Build history of the part. All positions in model axes, mm. A direction names the side the tool comes from. Give positions to 0.01 mm unless a question says otherwise; leave off trailing zeros. Order: outer loops, then holes, each group sorted by start corner. A loop starts at its lowest first (then second) coordinate and runs counter-clockwise, first axis right, second up. Notation, with made-up numbers: (62, 65.25) -> (89, 65.25) arc R18 ccw to (89, 89.25) -> close; hole circle Ø9 at (70, 83.5). An arc over 180 degrees is marked (long way). Write item = value, one per line. Start each with the question number.
from build123d import *

# Parameters (mm, degrees)
BOSS_EXTRUDE1_DEPTH = 76.2
FILLET1_R           = 127
CUT_EXTRUDE1_DEPTH  = 152.4
SKETCH4_R           = 38.1
CUT_EXTRUDE2_DEPTH  = 152.4
SKETCH5_R           = 330.2
SKETCH5_R_2         = 279.4
BOSS_EXTRUDE2_DEPTH = 76.2
CUT_EXTRUDE3_DEPTH  = 76.2
SKETCH7_R           = 279.4
CUT_EXTRUDE4_DEPTH  = 76.2
FILLET2_R           = 101.6
SKETCH10_R          = 19.05
CUT_EXTRUDE5_DEPTH  = 1983.041579978


with BuildPart() as part:
    # Sketch1 → Boss-Extrude1 (new, symmetric)
    with BuildSketch(Plane(origin=(0, 0, 0), x_dir=(1, 0, 0), z_dir=(0, 1, 0))):
        Polygon((666.144379946, 38.507212604), (1092.864379946, -322.007837556), (1913.344533237, -322.007837556), (1913.344533237, -398.207837556), (1064.984533237, -398.207837556), (638.264533237, -37.692787396), (-652.055466763, -37.692787396), (-652.055466763, 38.507212604), align=None)
    extrude(amount=BOSS_EXTRUDE1_DEPTH, both=True)

    # Fillet1
    fillet1_edges = [part.edges().sort_by_distance(p)[0] for p in [
        (666.144379946, 0, -38.507212604),
        (1092.864379946, 0, 322.007837556),
        (1064.984533237, 0, 398.207837556),
        (638.264533237, 0, 37.692787396),
    ]]
    fillet(fillet1_edges, radius=FILLET1_R)

    # Sketch3 → Cut-Extrude1 (cut)
    with BuildSketch(Plane.XY.offset(37.692787396)):
        with BuildLine():
            ThreePointArc((-652.055466763, -4.31e-07), (-629.737003641, 53.881536574), (-575.855466763, 76.2))
            Line((-575.855466763, 76.2), (-652.055466763, 76.2))
            Line((-652.055466763, 76.2), (-652.055466763, -4.31e-07))
        make_face()
        with BuildLine():
            ThreePointArc((-575.855466763, -76.2), (-629.737003336, -53.881536879), (-652.055466763, -4.31e-07))
            Line((-652.055466763, -4.31e-07), (-652.055466763, -76.2))
            Line((-652.055466763, -76.2), (-575.855466763, -76.2))
        make_face()
    extrude(amount=-CUT_EXTRUDE1_DEPTH, mode=Mode.SUBTRACT)

    # Sketch4 → Cut-Extrude2 (cut)
    with BuildSketch(Plane.XY.offset(37.692787396)):
        with Locations((-575.855466763, 0)):
            Circle(SKETCH4_R)
    extrude(amount=-CUT_EXTRUDE2_DEPTH, mode=Mode.SUBTRACT)

    # Sketch5 → Boss-Extrude2 (add)
    with BuildSketch(Plane.XY.offset(398.207837556)):
        with Locations((1583.144533237, 0)):
            Circle(SKETCH5_R)
        with Locations((1583.144533237, 0)):
            Circle(SKETCH5_R_2, mode=Mode.SUBTRACT)
    extrude(amount=-BOSS_EXTRUDE2_DEPTH)

    # Sketch6 → Cut-Extrude3 (cut)
    with BuildSketch(Plane.XY.offset(398.207837556)):
        with BuildLine():
            Line((1913.344533237, 76.2), (1904.431943511, 76.2))
            ThreePointArc((1904.431943511, 76.2), (1911.108817019, 38.359725806), (1913.344533237, 0))
            Line((1913.344533237, 0), (1913.344533237, 76.2))
        make_face()
        with BuildLine():
            Line((1913.344533237, -76.2), (1913.344533237, 0))
            ThreePointArc((1913.344533237, 0), (1911.108817019, -38.359725806), (1904.431943511, -76.2))
            Line((1904.431943511, -76.2), (1913.344533237, -76.2))
        make_face()
    extrude(amount=-CUT_EXTRUDE3_DEPTH, mode=Mode.SUBTRACT)

    # Sketch7 → Cut-Extrude4 (cut)
    with BuildSketch(Plane.XY.offset(398.207837556)):
        with Locations((1583.144533237, 0)):
            Circle(SKETCH7_R)
    extrude(amount=-CUT_EXTRUDE4_DEPTH, mode=Mode.SUBTRACT)

    # Fillet2
    fillet2_edges = [part.edges().sort_by_distance(p)[0] for p in [
        (1261.857122964, -76.2, 360.107837556),
        (1261.857122964, 76.2, 360.107837556),
    ]]
    fillet(fillet2_edges, radius=FILLET2_R)

    # Sketch10 → Cut-Extrude5 (cut, through all)
    with BuildSketch(Plane(origin=(0, 0, 0), x_dir=(1, 0, 0), z_dir=(0, 1, 0))):
        with Locations(Location((1583.144533237, -360.107837556, 0), (0, 0, 90))):
            Circle(SKETCH10_R)
    extrude(amount=CUT_EXTRUDE5_DEPTH, mode=Mode.SUBTRACT)


solid = part.part
(1) Wall check: line 1 (Y direction, x = 56, z = 18); line 2 (Z direction, x = -333, y = 40.5); line 3 (Z direction, x = 1411, y = -240). Give the ranges that are in metal, low to high. Write a range as [from, to].
(2) 3-axis set-ups, long thin cutter, end or side, ignore diameter. For faces 4 (the face through (-21, 1, 37.693)), 5 (the face through (1295, 2, 322.008)), 6 (the face through (-540.66, -14.59, 0.13)): which of +Z, -Z, +X, -X, +Y, -Y reach the whole face in a straight line?
(3) Cut at B-B, the plane x = -378. Give the cut face in (y, z).
(4) Mould opens along X. For faces 1 (the face through (1244.063, -92, 360.641)), 2 (the face through (-25, 1, -38.507)), 3 (the face through (1849.642, 83.924, 360.641)) say: released by +X, released by -X, zero draft, split by the parting line, or undercut.
(5) Cut at A-A, the plane y = 216. Give the cut face in (x, z), plus the area to 3 significant figures.
(6) Cut at C-C, the plane z = 226. Give the cut face in (x, y).
(7) Flat gauge pin, fed straight in: P1, Ø2, axis at y = -60.5, z = 236.5, coming from the -X side. Where does the tip first touch, or does it go through?
Results:
q1.line_1 = [-76.2, 76.2]
q1.line_2 = [-38.51, 37.69]
q1.line_3 = [322.01, 398.21]
q2.face_4 = +Z, -X, +Y, -Y
q2.face_5 = -Z, +X, +Y, -Y
q2.face_6 = +Z, -Z
q3.outline = (-76.2, -38.51) -> (76.2, -38.51) -> (76.2, 37.69) -> (-76.2, 37.69) -> close
q4.face_1 = released by -X
q4.face_2 = zero draft
q4.face_3 = undercut
q5.outline = (1333.39, 322.01) -> (1405.92, 322.01) -> (1405.92, 398.21) -> (1333.39, 398.21) -> close; (1760.37, 322.01) -> (1832.9, 322.01) -> (1832.9, 398.21) -> (1760.37, 398.21) -> close
q5.area = 11,100 mm2
q6.outline = (861.15, -76.2) -> (979.23, -76.2) -> (979.23, 76.2) -> (861.15, 76.2) -> close
q7.P1 = 872.4
